```python
from build123d import *

# Parameters (mm, degrees)
SCHIZZO1_R                   = 6
ESTRUSIONE_ESTRUSIONE1_DEPTH = 58
SCHIZZO2_R                   = 5.5
ESTRUSIONE_ESTRUSIONE2_DEPTH = 23
TAGLIO_ESTRUSIONE1_START     = -5.5
SCHIZZO3_W                   = 5
SCHIZZO3_H                   = 5
TAGLIO_ESTRUSIONE1_DEPTH     = 5
TAGLIO_ESTRUSIONE2_DEPTH     = 2.5
SMUSSO1_SIZE                 = 0.5


with BuildPart() as part:
    # Schizzo1 → Estrusione-Estrusione1 (new body)
    with BuildSketch(Plane(origin=(0, 0, 0), x_dir=(1, 0, 0), z_dir=(0, 1, 0))):
        with Locations(Location((0, 0, 0), (0, 0, 90))):
            Circle(SCHIZZO1_R)
    extrude(amount=ESTRUSIONE_ESTRUSIONE1_DEPTH)

    # Schizzo2 → Estrusione-Estrusione2 (add)
    with BuildSketch(Plane.XZ):
        with Locations(Location((0, 0, 0), (0, 0, 270))):
            Circle(SCHIZZO2_R)
    extrude(amount=ESTRUSIONE_ESTRUSIONE2_DEPTH)

    # Schizzo3 → Taglio-Estrusione1 (cut)
    with BuildSketch(Plane.XY.offset(TAGLIO_ESTRUSIONE1_START)):
        with Locations((0, 55.5)):
            Rectangle(SCHIZZO3_W, SCHIZZO3_H)
    extrude(amount=-TAGLIO_ESTRUSIONE1_DEPTH, mode=Mode.SUBTRACT)

    # Schizzo5 → Taglio-Estrusione2 (cut)
    with BuildSketch(Plane.XY.offset(5.5)):
        with BuildLine():
            Line((-2, -23), (-2, -9))
            ThreePointArc((-2, -9), (0, -7), (2, -9))
            Line((2, -9), (2, -23))
            ThreePointArc((2, -23), (0, -25), (-2, -23))
        make_face()
    extrude(amount=-TAGLIO_ESTRUSIONE2_DEPTH, mode=Mode.SUBTRACT)

    # Smusso1
    smusso1_edges = [part.edges().sort_by_distance(p)[0] for p in [
        (0, 0, 6),
        (0, 58, 6),
        (5.405049242, -23, -1.017567048),
    ]]
    chamfer(smusso1_edges, length=SMUSSO1_SIZE - 0.0001)  # a hair under: the kernel refuses the full size


solid = part.part
```
Here's how the part is built. I have some questions about the finished solid (model axes, mm). A direction names the side the tool comes from. Coordinates: 2 decimals unless noted, no trailing zeros. Order: outer loops, then holes, each group sorted by start corner. A loop starts at its lowest first (then second) coordinate and runs counter-clockwise, first axis right, second up.
1) Will these pins go through, and if not, where does the flat tip stop? pin 1 (5.5 mm diameter, centred on x = 1, y = 56.5, fed in from -Z); pin 2 (1.2 mm diameter, centred on x = -1, y = -16, fed in from +Z); pin 3 (1.1 mm diameter, centred on y = -15, z = 4, fed in from +X).
2) I need wall thicknesses on line 1 (Z direction, x = -0.25, y = 10.5); line 2 (X direction, y = 52.5, z = 5.5). Which ranges of each line are inside material? Lowest first, please.
3) Imagine slicing it at B-B on y = 39. List the corners of the cut face in (x, z) for me.
4) Which directions (+Z, -Z, +X, -X, +Y, -Y) give clear straight access to the entire face, cutting with the end or side of a thin tool? Please do faces 5 (the face through (0, 56, -5.5)), 6 (the face through (2, -16, 4)), 7 (the face through (-2.11, -11.09, -5.08)), 8 (the face through (0, 29, 6)).
5) We'd pull the mould along X, two halves only. Please class faces 1 (the face through (-2, -16, 4)), 2 (the face through (0, 58, 0)), 3 (the face through (-0.199, -22.865, -5.132)), 4 (the face through (0, -7, 4)): +X half, -X half, draft (parallel to the pull), parting line (faces both ways), or undercut.
Response values:
1. pin 1: stops at z = -5.5
1. pin 2: stops at z = 3
1. pin 3: stops at x = 4.28
2. line 1: z = -5.99 to 5.99
2. line 2: x = -2.4 to 2.4
3. outline: circle Ø12 at (0, 0)
4. face 5: -Z, +X, -X, +Y
4. face 6: +Z, -Y
4. face 7: -Y
4. face 8: +Y, -Y
5. face 1: undercut
5. face 2: draft
5. face 3: parting line
5. face 4: undercut
